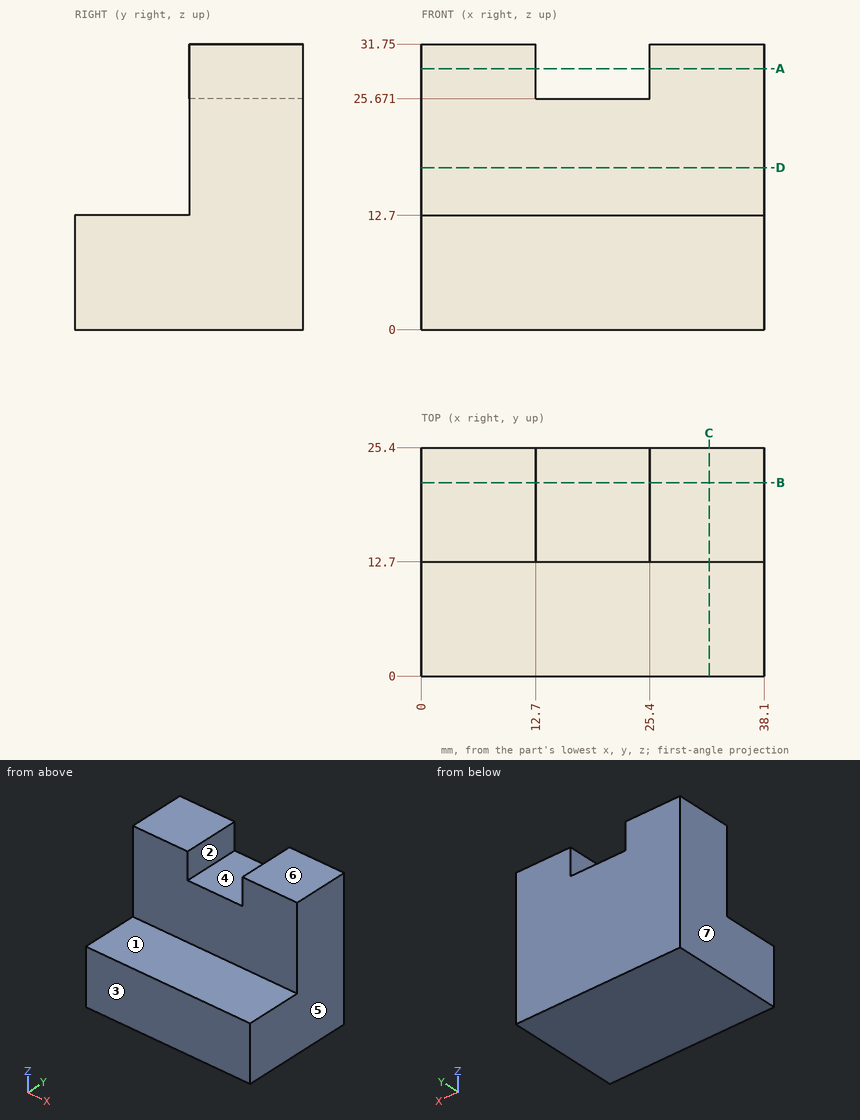
Study the drawing (mm; zero at the part's minimum x, y, z) and answer. A direction names the side the tool comes from. Coordinates: 2 decimals unless noted, no trailing zeros. Loops run counter-clockwise (first coordinate to the right, second up) from the corner with the lowest first, then second, coordinate; pieces in that order, holes last. Notation, with made-up numbers: (86.25, 83) -> (137.25, 83) arc R16 ccw to (137.25, 99) -> close; hole circle Ø1 at (75.5, -4.5). An arc over 180 degrees is marked (long way). Answer in a Markdown table with one row per item. Add a question column.
1. The part is cut by section A-A, the plane z = 29. Write down the section's boundary in (x, y).
2. Flat-ended cylindrical pins translate along their axes: P1, Ø3, axis at x = 19.5, y = 9, coming from the +Z side; P2, Ø2, axis at y = 10, z = 16.5, coming from the +X side; P3, Ø6, axis at x = 21.5, y = 10, coming from the +Z side. Find the tip coordinate at first contact, or state that the pin passes through.
3. Determine the mould class of the marked faces 4, 5, 6 and 7 for opening direction X: +X half, -X half, draft (parallel to the pull), parting line (faces both ways), or undercut.
4. For the marked faces 1, 2 and 3, determine the directions among +Z, -Z, +X, -X, +Y, -Y from which every point of the face is accessible in a straight line to the end or side of a thin tool.
5. The part is cut by section D-D, the plane z = 18. Write down the section's boundary in (x, y), then the cut area to 3 significant figures.
6. The part is cut by section B-B, the plane y = 21.5. Write down the section's boundary in (x, z), then the cut area to 3 significant figures.
7. Consider line 1 (X direction, y = 23.5, z = 28); line 2 (Z direction, x = 24, y = 22.75); line 3 (Z direction, x = 28.5, y = 1.75). Determine where each line is inside the solid, lowest interval first. Write a range as [from, to].
8. The part is cut by section C-C, the plane x = 32. Write down the section's boundary in (y, z).
Answer below:
| question | item | result |
|---|---|---|
| 1 | outline | (0, 12.7) -> (12.7, 12.7) -> (12.7, 25.4) -> (0, 25.4) -> close; (25.4, 12.7) -> (38.1, 12.7) -> (38.1, 25.4) -> (25.4, 25.4) -> close |
| 2 | P1 | z = 12.7 |
| 2 | P2 | through |
| 2 | P3 | z = 25.67 |
| 3 | face 4 | undercut |
| 3 | face 5 | +X half |
| 3 | face 6 | draft |
| 3 | face 7 | -X half |
| 4 | face 1 | +Z, +X, -X, -Y |
| 4 | face 2 | +Z, +Y, -Y |
| 4 | face 3 | +Z, -Z, +X, -X, -Y |
| 5 | outline | (0, 12.7) -> (38.1, 12.7) -> (38.1, 25.4) -> (0, 25.4) -> close |
| 5 | area | 484 mm2 |
| 6 | outline | (0, 0) -> (38.1, 0) -> (38.1, 31.75) -> (25.4, 31.75) -> (25.4, 25.67) -> (12.7, 25.67) -> (12.7, 31.75) -> (0, 31.75) -> close |
| 6 | area | 1,130 mm2 |
| 7 | line 1 | [0, 12.7], [25.4, 38.1] |
| 7 | line 2 | [0, 25.67] |
| 7 | line 3 | [0, 12.7] |
| 8 | outline | (0, 0) -> (25.4, 0) -> (25.4, 31.75) -> (12.7, 31.75) -> (12.7, 12.7) -> (0, 12.7) -> close |
